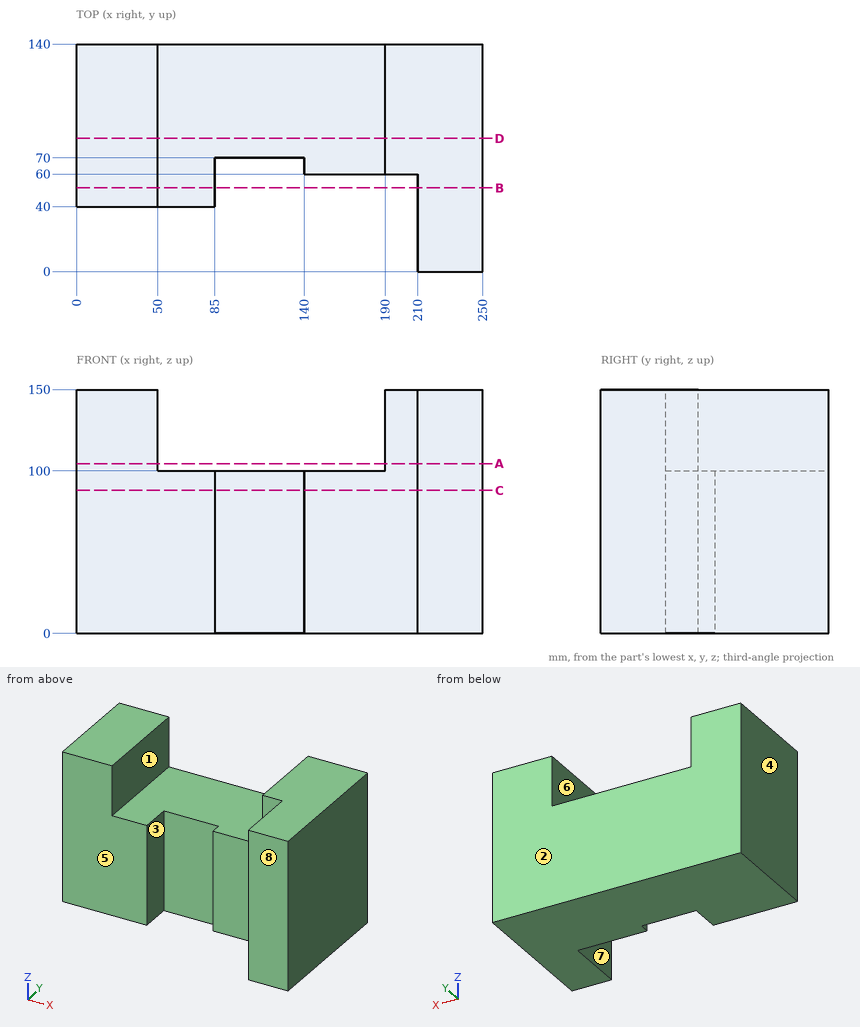
The figure shows three views and two pictorial views of one solid part (mm, origin at its lowest corner). Answer the questions. A direction names the side the tool comes from. Give positions to 0.01 mm unless a question says otherwise; leave off trailing zeros. Order: outer loops, then holes, each group sorted by start corner. A loop starts at its lowest first (then second) coordinate and runs counter-clockwise, first axis right, second up. Notation, with made-up numbers: (86.5, 32.25) -> (90.5, 32.25) arc R32 cw to (90.5, 61.25) -> close; hole circle Ø1 at (12, -21). An arc over 180 degrees is marked (long way). One line per item, written item: value.
1) Find the intervals of material crossed by line 1 (X direction, y = 61.5, z = 42); line 2 (X direction, y = 61, z = 125); line 3 (Z direction, x = 174.5, y = 94.5), in increasing order.
Reported:
line 1: x = 0 to 85, 140 to 250
line 2: x = 0 to 50, 190 to 250
line 3: z = 0 to 100
2) A tool of negligible diameter and unlimited length cuts with its end or side. For the marked faces 5, 6, 7 and 8, from which of +Z, -Z, +X, -X, +Y, -Y can it reach the whole face along a straight path? Write none if from no direction.
Reported:
face 5: +Z, -Z, -X, -Y
face 6: +Z, +Y, -Y
face 7: +Z, -Z, -Y
face 8: +Z, -Z, +X, -X, -Y
3) Determine the mould class of the marked faces 1, 2, 3 and 4 for opening direction X: pulls with the +X half, pulls with the -X half, needs draft (parallel to the pull), parting line crosses it, or undercut.
Reported:
face 1: undercut
face 2: needs draft
face 3: undercut
face 4: pulls with the -X half
4) Find section C-C, the plane z = 88. Determine the outline of the cut face in (x, y).
Reported:
outline: (0, 40) -> (85, 40) -> (85, 70) -> (140, 70) -> (140, 60) -> (210, 60) -> (210, 0) -> (250, 0) -> (250, 140) -> (0, 140) -> close
5) Find section D-D, the plane y = 82. Determine the outline of the cut face in (x, z).
Reported:
outline: (0, 0) -> (250, 0) -> (250, 150) -> (190, 150) -> (190, 100) -> (50, 100) -> (50, 150) -> (0, 150) -> close
6) Find section B-B, the plane y = 51.5. Determine the outline of the cut face in (x, z), plus the area to 3 significant figures.
Reported:
outline: (0, 0) -> (85, 0) -> (85, 100) -> (50, 100) -> (50, 150) -> (0, 150) -> close; (210, 0) -> (250, 0) -> (250, 150) -> (210, 150) -> close
area: 17,000 mm^2
7) Find section A-A, the plane z = 104.5. Determine the outline of the cut face in (x, y).
Reported:
outline: (0, 40) -> (50, 40) -> (50, 140) -> (0, 140) -> close; (190, 60) -> (210, 60) -> (210, 0) -> (250, 0) -> (250, 140) -> (190, 140) -> close
8) Flat-ended cylindrical pins translate along their axes: P1, Ø1, axis at y = 87, z = 98, coming from the -X side; P2, Ø4, axis at x = 114.5, z = 99.5, coming from the -Y side; P3, Ø4, axis at x = 61, z = 46, coming from the -Y side. Find the tip coordinate at first contact, or state that the pin passes through.
Reported:
P1: stops at x = 0
P2: stops at y = 70
P3: stops at y = 40
